Verification items for the finished model (mm, model axes). A direction names the side the tool comes from. Give positions to 0.01 mm unless a question says otherwise; leave off trailing zeros. Loops run counter-clockwise (first coordinate to the right, second up) from the corner with the lowest first, then second, coordinate; pieces in that order, holes last. Notation, with made-up numbers: (-37.5, -14) -> (-3.5, -14) arc R25 ccw to (-3.5, 18) -> close; hole circle Ø4 at (-3.75, 44). An arc over 180 degrees is marked (long way). Answer in a Markdown table with one row per item. Add a question column.
Q1. Material ranges on probe 1 along Y at (x, z) = (-11.7, -5.6) (3 decimals); probe 2 along X at (y, z) = (0.9, 0) (3 decimals); probe 3 along Y at (x, z) = (7.7, 5.65) (3 decimals), recorded low to high.
Q2. Release check for a two-part mould opening along X. For faces 4 (the face through (1, 1, -6.65)), 5 (the face through (10, 1, 0)), 6 (the face through (-13.399, 7.285, -5.486)), 7 (the face through (2, 0, 0)) record: pulls with the +X half, pulls with the -X half, needs draft (parallel to the pull), parting line crosses it, or undercut.
Q3. Section check D-D on y = 6.5. Enter the section's corners in (x, z), and give its area (3 significant figures).
Q4. Section check C-C on x = -11.7. Enter the section's corners in (y, z) (3 decimals), and give its area (3 significant figures).
Q5. Set-up check for faces 1 (the face through (-5.7, 6, -5)), 2 (the face through (-9, 7, -4.5)), 3 (the face through (-0.55, 1, 0)): record each of +Z, -Z, +X, -X, +Y, -Y from which the full face is reachable in a straight line by a thin tool's end or side.
Q6. Gauge pin test, flat ends, axial feed: P1, Ø1, axis at y = 3, z = 6, coming from the -X side; P2, Ø6, axis at y = 7, z = 4.5, coming from the +X side; P3, Ø2, axis at y = 1.5, z = 1, coming from the -X side; P4, Ø2, axis at x = 7.7, y = 9, coming from the -Z side. Record the tip position at first contact, or that the pin passes through.
Q7. Section check A-A on y = 9. Enter the section's corners in (x, z) (3 decimals).
Q8. Section check B-B on z = 0. Enter the section's corners in (x, y) (3 decimals).
```python
from build123d import *

# Parameters (mm, degrees)
CROQUIS1_R              = 1.125
CROQUIS1_R_2            = 3.25
CROQUIS1_W              = 2.3
CROQUIS1_H              = 13.3
SALIENTE_EXTRUIR1_DEPTH = 2
CROQUIS2_W              = 4
CROQUIS2_H              = 2
SALIENTE_EXTRUIR2_DEPTH = 9
CROQUIS3_R              = 1.125
CORTAR_EXTRUIR1_DEPTH   = 13
CROQUIS5_W              = 2
CROQUIS5_H              = 4
SALIENTE_EXTRUIR3_DEPTH = 4
CROQUIS6_R              = 1.125
CORTAR_EXTRUIR3_DEPTH   = 25.102696945
REDONDEO2_R             = 1


with BuildPart() as part:
    # Croquis1 → Saliente-Extruir1 (new body)
    with BuildSketch(Plane(origin=(0, 0, 0), x_dir=(1, 0, 0), z_dir=(0, 1, 0))):
        with BuildLine():
            Line((-5, -10), (7.32626704, -10))
            ThreePointArc((7.32626704, -10), (9.216881747, -9.216881747), (10, -7.32626704))
            Line((10, -7.32626704), (10, 7))
            ThreePointArc((10, 7), (9.121320344, 9.121320344), (7, 10))
            Line((7, 10), (-5, 10))
            ThreePointArc((-5, 10), (-8.535533906, 8.535533906), (-10, 5))
            Line((-10, 5), (-10, -5))
            ThreePointArc((-10, -5), (-8.535533906, -8.535533906), (-5, -10))
        make_face()
        with Locations(Location((7.75, 0, 0), (0, 0, 270))):
            Circle(CROQUIS1_R, mode=Mode.SUBTRACT)
        with Locations(Location((-5.25, 0, 0), (0, 0, 270))):
            Circle(CROQUIS1_R_2, mode=Mode.SUBTRACT)
        with Locations((0.6, 0)):
            Rectangle(CROQUIS1_W, CROQUIS1_H, mode=Mode.SUBTRACT)
    extrude(amount=SALIENTE_EXTRUIR1_DEPTH)

    # Croquis2 → Saliente-Extruir2 (add)
    with BuildSketch(Plane(origin=(0, 2, 0), x_dir=(1, 0, 0), z_dir=(0, 1, 0))):
        with Locations((-7.7, 5.5)):
            Rectangle(CROQUIS2_W, CROQUIS2_H)
        with Locations((-7.7, -5.5)):
            Rectangle(CROQUIS2_W, CROQUIS2_H)
        with Locations((7.7, -5.5)):
            Rectangle(CROQUIS2_W, CROQUIS2_H)
    extrude(amount=SALIENTE_EXTRUIR2_DEPTH)

    # Croquis3 → Cortar-Extruir1 (cut)
    with BuildSketch(Plane.XY.offset(6.5)):
        with Locations((7.7, 9)):
            Circle(CROQUIS3_R)
    extrude(amount=-CORTAR_EXTRUIR1_DEPTH, mode=Mode.SUBTRACT)

    # Croquis5 → Saliente-Extruir3 (add)
    with BuildSketch(Plane.ZY.offset(9.7)):
        with Locations((5.5, 9)):
            Rectangle(CROQUIS5_W, CROQUIS5_H)
        with Locations((-5.5, 9)):
            Rectangle(CROQUIS5_W, CROQUIS5_H)
    extrude(amount=SALIENTE_EXTRUIR3_DEPTH)

    # Croquis6 → Cortar-Extruir3 (cut, through all)
    with BuildSketch(Plane.XY.offset(6.5)):
        with Locations((-11.7, 9)):
            Circle(CROQUIS6_R)
    extrude(amount=-CORTAR_EXTRUIR3_DEPTH, mode=Mode.SUBTRACT)

    # Redondeo2
    redondeo2_edges = [part.edges().sort_by_distance(p)[0] for p in [
        (-13.7, 11, -5.5),
        (-13.7, 7, -5.5),
        (-5.7, 11, -5.5),
        (-5.7, 11, 5.5),
        (5.7, 11, 5.5),
        (9.7, 11, 5.5),
        (-13.7, 7, 5.5),
        (-13.7, 11, 5.5),
    ]]
    fillet(redondeo2_edges, radius=REDONDEO2_R)


solid = part.part
```
Taken from the geometry:
| question | item | result |
|---|---|---|
| 1 | probe 1 | y = 7 to 7.875, 10.125 to 11 |
| 1 | probe 2 | x = -10 to -8.5, -2 to -0.55, 1.75 to 6.625, 8.875 to 10 |
| 1 | probe 3 | y = 0 to 7.875, 10.125 to 11 |
| 2 | face 4 | undercut |
| 2 | face 5 | pulls with the +X half |
| 2 | face 6 | pulls with the -X half |
| 2 | face 7 | needs draft |
| 3 | outline | (-9.7, -6.5) -> (-5.7, -6.5) -> (-5.7, -4.5) -> (-9.7, -4.5) -> close; (-9.7, 4.5) -> (-5.7, 4.5) -> (-5.7, 6.5) -> (-9.7, 6.5) -> close; (5.7, 4.5) -> (9.7, 4.5) -> (9.7, 6.5) -> (5.7, 6.5) -> close |
| 3 | area | 24.0 mm² |
| 4 | outline | (7, -6.5) -> (7.875, -6.5) -> (7.875, -4.5) -> (7, -4.5) -> close; (7, 4.5) -> (7.875, 4.5) -> (7.875, 6.5) -> (7, 6.5) -> close; (10.125, -6.5) -> (11, -6.5) -> (11, -4.5) -> (10.125, -4.5) -> close; (10.125, 4.5) -> (11, 4.5) -> (11, 6.5) -> (10.125, 6.5) -> close |
| 4 | area | 7.00 mm² |
| 5 | face 1 | +Z, -Z, +X, +Y |
| 5 | face 2 | +X, -X, +Y |
| 5 | face 3 | +Y, -Y |
| 6 | P1 | stops at x = -9.7 |
| 6 | P2 | stops at x = 9.7 |
| 6 | P3 | stops at x = -10 |
| 6 | P4 | passes through |
| 7 | outline | (-13.7, -6.5) -> (-12.825, -6.5) -> (-12.825, -4.5) -> (-13.7, -4.5) -> close; (-13.7, 4.5) -> (-12.825, 4.5) -> (-12.825, 6.5) -> (-13.7, 6.5) -> close; (-10.575, -6.5) -> (-5.7, -6.5) -> (-5.7, -4.5) -> (-10.575, -4.5) -> close; (-10.575, 4.5) -> (-5.7, 4.5) -> (-5.7, 6.5) -> (-10.575, 6.5) -> close; (5.7, 4.5) -> (6.575, 4.5) -> (6.575, 6.5) -> (5.7, 6.5) -> close; (8.825, 4.5) -> (9.7, 4.5) -> (9.7, 6.5) -> (8.825, 6.5) -> close |
| 8 | outline | (-10, 0) -> (-8.5, 0) -> (-8.5, 2) -> (-10, 2) -> close; (-2, 0) -> (-0.55, 0) -> (-0.55, 2) -> (-2, 2) -> close; (1.75, 0) -> (6.625, 0) -> (6.625, 2) -> (1.75, 2) -> close; (8.875, 0) -> (10, 0) -> (10, 2) -> (8.875, 2) -> close |
